Could you check a few things on this model? Use its own coordinates, in mm. A direction names the side the tool comes from. Coordinates: 2 decimals unless noted, no trailing zeros. Write each loop counter-clockwise with the first axis right and the second up, starting at its lowest first coordinate (ties: lowest second). Pieces come first, ordered by that corner, then holes.
Item 1: I want a section at B-B on z = -4.5. State how many separate pieces and enclosed holes the cut face has, then the cut area to 3 significant figures.
Item 2: If I drill on probe 1 along X at (y, z) = (14, -30); probe 2 along Y at (x, z) = (25.5, -13.5); probe 3 along Y at (x, z) = (-12.5, -21), over which ranges is the centre line in solid material (lowest first)?
Item 3: Thinking about a two-plate mould opening in Y: for faces 5 (the conical face through (35.38, 36.08, -4.61)), 6 (the conical face through (-28.923, 9.598, -27.66)), 7 (the conical face through (34.938, 25.724, -4.769)), which applies, +Y half, -Y half, draft (parallel to the pull), parting line (faces both ways), or undercut?
Item 4: Which directions (+Z, -Z, +X, -X, +Y, -Y) give clear straight access to the entire face, cutting with the end or side of a thin tool? Please do faces 1 (the conical face through (15.09, -6.973, -11.884)), 2 (the conical face through (14.94, 12.11, -11.94)), 3 (the conical face through (20.028, 38.466, -10.113)), 4 (the conical face through (-13.62, 24.01, -22.17)).
Item 5: For P1, Ø1, axis at y = 39.5, z = -29.5, coming from the +X side; P2, Ø3.5, axis at x = 19, z = -15, coming from the -Y side; P3, Ø8, axis at x = -13.5, z = -41.5, coming from the -Y side, each with a flat end and sliding along its axis, tell me the tip position at first contact or that it passes through.
Item 6: I want a section at C-C on y = 1. Please give me the cut outline in (x, z), then the cut area to 3 significant figures.
Item 7: I want a section at A-A on y = 44. Please give me the cut outline in (x, z).
from build123d import *

# Parameters (mm, degrees)
F1_ANGLE = 40


with BuildPart() as f1:
    # F0 (on Top) → F1 (revolve)
    with BuildSketch(Plane.XY):
        Polygon((28.799957, 21.561632), (28.799957, 12.819916), (35.130166, 21.561632), (31.819634, 23.958914), (36.335919, 27.439682), (36.335919, 32.262698), (32.869376, 39.798658), (26.38845, 46.430305), (19.756803, 49.896847), (16.742419, 49.896847), (15.385945, 47.636058), (16.742419, 42.210165), (19.756803, 34.824926), (22.780804, 30.966716), (24.12766, 29.248312), align=None)
        Polygon((35.130166, 21.561632), (28.799957, 12.819916), (28.799957, 21.561632), (24.12766, 29.248312), (22.780804, 30.966716), (22.017591, 23.520982), (16.667058, 28.871514), (14.180192, 31.35838), (11.870201, 31.595162), (5.361195, 32.262357), (1.154359, 32.693573), (-0.653343, 36.710685), (-2.549643, 34.674205), (-5.52113, 34.978793), (-2.549643, 33.016294), (-7.975536, 33.016294), (-4.207555, 31.35838), (-8.431453, 29.457625), (-13.552147, 25.932489), (-16.19102, 26.202983), (-19.430198, 20.657316), (-21.540266, 13.272074), (-21.540266, 6.489708), (-20.952175, 3.67613), (-20.183794, 0), (-18.073725, -2.633195), (-15.963655, -5.266391), (-7.824816, -8.431495), (0, -9.233566), (8.000703, -9.233566), (16.128225, -5.576178), (22.16831, -1.347692), (22.16831, 0), (26.23773, 4.379639), (26.539169, 7.394024), (31.060746, 11.162004), (34.469465, 16.161462), align=None)
        Polygon((-17.773023, 10.257689), (-14.139653, 14.920566), (-11.414627, 14.920566), (-10.262036, 13.024369), (-8.856477, 10.711998), (-8.783638, 9.730172), (-7.640627, 7.849735), (-11.959632, 3.657121), (-17.415215, 5.434674), align=None, mode=Mode.SUBTRACT)
        Polygon((14.745632, 3.657121), (11.112262, 5.736113), (15.201996, 5.736113), align=None, mode=Mode.SUBTRACT)
        Polygon((6.794949, 17.492212), (9.884694, 14.262024), (10.110772, 14.02567), (9.884694, 13.583343), (6.644229, 7.243304), (3.026968, 5.736113), (-3.152521, 7.092585), (-5.865466, 10.257689), (-5.865466, 14.929986), (-4.358274, 16.286459), (-1.796047, 18.547246), (3.394514, 19.138865), align=None, mode=Mode.SUBTRACT)
        Polygon((13.655621, 11.105528), (11.657268, 13.648886), (11.657268, 18.735604), (14.563963, 21.6423), (18.924005, 21.6423), (21.830701, 18.735605), (21.830701, 12.377207), (17.222896, 10.303694), (13.922315, 11.990658), align=None, mode=Mode.SUBTRACT)
        Polygon((-24.554653, 0), (-18.073725, -2.633195), (-20.183794, 0), (-20.952175, 3.67613), (-21.540266, 6.489708), (-21.540266, 13.272074), (-23.801055, 20.205159), (-27.232317, 25.628765), (-28.624071, 37.839308), (-30.305653, 40.497292), (-34.044402, 38.131959), (-36.310751, 32.111976), (-38.270105, 23.671702), (-36.91363, 14.628547), (-31.764652, 6.489844), align=None)
    revolve(axis=Axis((48.242737, 22.056726, 0), (0, -1, 0)), revolution_arc=F1_ANGLE)


solid = f1.part
Response values:
1. separate pieces: 1
1. enclosed holes: 4
1. area: 2,190 mm2
2. probe 1: x = -31.03 to -15.03, -14.53 to -7.27, -2.67 to 3.21
2. probe 2: y = -1.61 to 12.36, 18.77 to 23.74, 32.22 to 48.83
2. probe 3: y = -5.19 to 4.98, 12.5 to 26.19
3. face 5: +Y half
3. face 6: -Y half
3. face 7: undercut
4. face 1: +Z, +X, -Y
4. face 2: none
4. face 3: -Z
4. face 4: +Y
5. P1: stops at x = -23.48
5. P2: stops at y = -6.7
5. P3: stops at y = -0.98
6. outline: (-25.67, 0) arc R73.91 ccw to (-8.37, -47.51) - (28.98, -16.16) arc R25.15 cw to (23.1, 0) - close
6. area: 1,690 mm2
7. outline: (16.29, 0) arc R31.95 ccw to (23.77, -20.54) - (33.32, -12.52) arc R19.48 cw to (28.76, 0) - close
